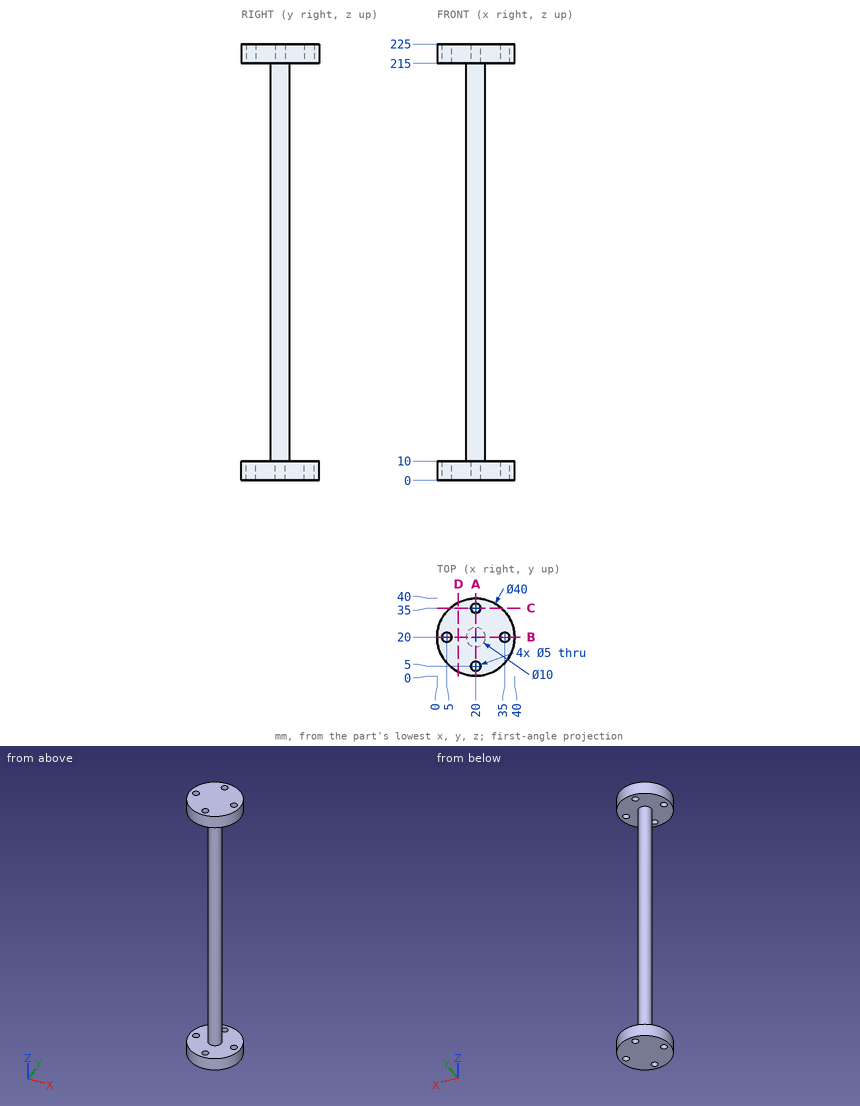
For this review, use the dimensioned drawing (mm, ordinates from the lowest corner) and the shaded views. Round coordinates to 2 decimals unless told otherwise and drop trailing zeros. Order: outer loops, then holes, each group sorted by start corner. A loop starts at its lowest first (then second) coordinate and runs counter-clockwise, first axis right, second up. Notation, with made-up numbers: (42, -28.75) -> (64, -28.75) arc R27 ccw to (64, 5.25) -> close; hole circle Ø2 at (49, -19). An arc over 180 degrees is marked (long way). Write item = value, one per line. Start each with the question number.
Item 1: Consider section C-C on y = 35. Write out the cut boundary in (x, z), plus the area to 3 significant figures.
Item 2: Consider section A-A on x = 20. Write out the cut boundary in (y, z).
Item 3: Clearance check with flat-ended pins moving along their axes: pin 1 Ø8 at (y, z) = (25.5, 61) entering from +X; pin 2 Ø8 at (y, z) = (13.5, 160.5) entering from -X; pin 3 Ø12 at (x, z) = (17, 177) entering from -Y; pin 4 Ø8 at (x, y) = (35, 20) entering from +Z. State where each tip first meets the part, or that it passes through.
Item 4: Consider section D-D on x = 11. Write out the cut boundary in (y, z), plus the area to 3 significant figures.
Item 5: For line 1 along Y through (x, z) = (20, 7.5); line 2 along Z through (x, y) = (19, 38.5); line 3 along X through (y, z) = (19.5, 154.5), list the stretches that pass through material, from the lowest coordinate up.
Conclusion:
q1.outline = (6.77, 0) -> (17.5, 0) -> (17.5, 10) -> (6.77, 10) -> close; (6.77, 215) -> (17.5, 215) -> (17.5, 225) -> (6.77, 225) -> close; (22.5, 0) -> (33.23, 0) -> (33.23, 10) -> (22.5, 10) -> close; (22.5, 215) -> (33.23, 215) -> (33.23, 225) -> (22.5, 225) -> close
q1.area = 429 mm2
q2.outline = (0, 0) -> (2.5, 0) -> (2.5, 10) -> (0, 10) -> close; (0, 215) -> (2.5, 215) -> (2.5, 225) -> (0, 225) -> close; (7.5, 0) -> (32.5, 0) -> (32.5, 10) -> (25, 10) -> (25, 215) -> (32.5, 215) -> (32.5, 225) -> (7.5, 225) -> (7.5, 215) -> (15, 215) -> (15, 10) -> (7.5, 10) -> close; (37.5, 0) -> (40, 0) -> (40, 10) -> (37.5, 10) -> close; (37.5, 215) -> (40, 215) -> (40, 225) -> (37.5, 225) -> close
q3.pin_1 = 24.77
q3.pin_2 = 15.67
q3.pin_3 = 15
q3.pin_4 = 225
q4.outline = (2.14, 0) -> (37.86, 0) -> (37.86, 10) -> (2.14, 10) -> close; (2.14, 215) -> (37.86, 215) -> (37.86, 225) -> (2.14, 225) -> close
q4.area = 714 mm2
q5.line_1 = 0 to 2.5, 7.5 to 32.5, 37.5 to 40
q5.line_2 = 0 to 10, 215 to 225
q5.line_3 = 15.03 to 24.97
